from build123d import *

# Parameters (mm, degrees)
F1_DEPTH = 9.525
F3_DEPTH = 4.445


with BuildPart() as f1:
    # F0 (on Front) → F1 (new body)
    with BuildSketch(Plane.XZ):
        with BuildLine():
            ThreePointArc((-5.707243, -7.21562), (-9.19628, -0.257349), (-6.101839, 6.885154))
            ThreePointArc((-6.101839, 6.885154), (-5.88147, 7.779725), (-6.639719, 8.303058))
            Line((-6.639719, 8.303058), (-6.639719, 7.998258))
            ThreePointArc((-6.639719, 7.998258), (-6.166454, 7.671617), (-6.303998, 7.113266))
            ThreePointArc((-6.303998, 7.113266), (-9.500428, -0.284281), (-5.8674, -7.47747))
            Line((-5.8674, -7.47747), (-5.8674, -9.920767))
            Line((-5.8674, -9.920767), (-5.8674, -10.867245))
            Line((-5.8674, -10.867245), (5.8674, -10.867245))
            Line((5.8674, -10.867245), (5.8674, -7.47747))
            ThreePointArc((5.8674, -7.47747), (9.502004, -0.225537), (6.215559, 7.190673))
            ThreePointArc((6.215559, 7.190673), (6.072203, 7.750216), (6.54657, 8.079787))
            Line((6.54657, 8.079787), (6.54657, 8.384587))
            ThreePointArc((6.54657, 8.384587), (5.786557, 7.856561), (6.016236, 6.960079))
            ThreePointArc((6.016236, 6.960079), (9.197695, -0.200486), (5.707243, -7.21562))
            ThreePointArc((5.707243, -7.21562), (5.600662, -7.34845), (5.5626, -7.514445))
            Line((5.5626, -7.514445), (5.5626, -10.562445))
            Line((5.5626, -10.562445), (-5.5626, -10.562445))
            Line((-5.5626, -10.562445), (-5.5626, -9.920767))
            Line((-5.5626, -9.920767), (-5.5626, -7.514445))
            ThreePointArc((-5.5626, -7.514445), (-5.600662, -7.34845), (-5.707243, -7.21562))
        make_face()
    extrude(amount=F1_DEPTH)

    # F2 (on Right) → F3 (join, symmetric)
    with BuildSketch(Plane.YZ):
        with BuildLine():
            Line((0, -10.562445), (0, -10.867245))
            Line((0, -10.867245), (3.1623, -10.867245))
            ThreePointArc((3.1623, -10.867245), (3.476609, -10.737054), (3.6068, -10.422745))
            Line((3.6068, -10.422745), (3.6068, 3.748756))
            ThreePointArc((3.6068, 3.748756), (3.617336, 3.844964), (3.648446, 3.93661))
            Line((3.648446, 3.93661), (4.455377, 5.667079))
            Line((4.455377, 5.667079), (4.179134, 5.795893))
            Line((4.179134, 5.795893), (3.372204, 4.065424))
            ThreePointArc((3.372204, 4.065424), (3.319761, 3.910935), (3.302, 3.748756))
            Line((3.302, 3.748756), (3.302, -10.562445))
            Line((3.302, -10.562445), (0, -10.562445))
        make_face()
    extrude(amount=F3_DEPTH, both=True)

    # F4 (on Right) → F5 (revolve)
    with BuildSketch(Plane.YZ):
        with BuildLine():
            Line((3.302, -1.088245), (2.032, -1.088245))
            ThreePointArc((2.032, -1.088245), (2.374146, -2.316276), (3.302, -3.190469))
            Line((3.302, -3.190469), (3.302, -1.088245))
        make_face()
    revolve(axis=Axis((0, 2.667, -1.088245), (0, -1, 0)))


solid = f1.part
Can you work these out from the model? Positions are in its coordinate system, mm. A direction names the side the tool comes from. Give positions to 0.01 mm unless a question says otherwise; leave off trailing zeros. Loops run counter-clockwise (first coordinate to the right, second up) from the corner with the lowest first, then second, coordinate; pieces in that order, holes last. Notation, with made-up numbers: M 31.5,65 L 73.5,65 A19 ccw 73.5,102 Z; hole C 58,89 d5. An arc over 180 degrees is marked long. One line per item, written item: value. Start each with the question number.
1) Thinking about a two-plate mould opening in X: for faces 6 (the face through (0.06, 3.78, 4.94)), 7 (the face through (9.5, -4.7, -0.3)), 8 (the face through (0, -3, -10.562)), 9 (the face through (-5.867, -5, -9)), which applies, +X half, -X half, draft (parallel to the pull), parting line (faces both ways), or undercut?
2) I'm going to push flat-ended pins straight in: pin 1 (8 mm diameter, centred on y = -1.5, z = -6.5, fed in from +X); pin 2 (5.5 mm diameter, centred on x = -6.5, z = -1, fed in from +Y); pin 3 (2.5 mm diameter, centred on y = -3, z = -9, fed in from -X); pin 4 (1.3 mm diameter, centred on y = 1.5, z = -3.5, fed in from +X). Where does each tip first touch, or does it pass through?
3) If we section it at B-B, the plane z = 6.5: Write out the boundary of the cut face in (x, y) (3 decimals), and give its area (3 significant figures).
4) On a 3-axis mill with a long thin cutter (end or side, diameter ignored), from which of +Z, -Z, +X, -X, +Y, -Y can I reach the whole of each face in a straight line? I mean faces 1 (the face through (6.07, -4.7, 7.74)), 2 (the face through (-5.563, -5, -9)), 3 (the face through (-9.503, -4.696, -0.168)), 4 (the face through (0, 3.607, -3)), 5 (the face through (9.2, -4.7, -0.1)). Say none if no direction works.
5) If I drill on line 1 (X direction, y = -8.75, z = -9.5); line 2 (Z direction, x = 6.5, y = -7.75); line 3 (X direction, y = -2.5, z = 3.5), over which ranges is the centre line in solid material (lowest first)? Write a range as [from, to].
6) If we section it at A-A, the plane z = -8.75: Write out the boundary of the cut face in (x, y) (3 decimals), and give its area (3 significant figures).
7) If we section it at D-D, the plane y = -8.25: Write out the boundary of the cut face in (x, z).
Completed:
1. face 6: draft
1. face 7: +X half
1. face 8: undercut
1. face 9: -X half
2. pin 1: stops at x = 9.17
2. pin 2: stops at y = 3.61
2. pin 3: stops at x = -5.87
2. pin 4: passes through
3. outline: M -6.935,-9.525 L -6.511,-9.525 L -6.511,0 L -6.935,0 Z; M 6.511,-9.525 L 6.935,-9.525 L 6.935,0 L 6.511,0 Z
3. area: 8.08 mm^2
4. face 1: +X, +Y, -Y
4. face 2: +Z, +Y, -Y
4. face 3: -X, +Y, -Y
4. face 4: -Z, +X, -X, +Y
4. face 5: +Y, -Y
5. line 1: x = [-5.87, -5.56], [5.56, 5.87]
5. line 2: z = [-6.93, -6.51], [6.51, 6.93], [8.08, 8.38]
5. line 3: x = [-8.84, -8.51], [8.51, 8.84]
6. outline: M -5.867,-9.525 L -5.563,-9.525 L -5.563,0 L -5.867,0 Z; M -4.445,3.302 L 4.445,3.302 L 4.445,3.607 L -4.445,3.607 Z; M 5.563,-9.525 L 5.867,-9.525 L 5.867,0 L 5.563,0 Z
6. area: 8.52 mm^2
7. outline: M -6.64,8 A0.51 cw -6.3,7.11 A9.5 ccw -5.87,-7.48 L -5.87,-10.87 L 5.87,-10.87 L 5.87,-7.48 A9.5 ccw 6.22,7.19 A0.51 cw 6.55,8.08 L 6.55,8.38 A0.81 ccw 6.02,6.96 A9.2 cw 5.71,-7.22 A0.38 ccw 5.56,-7.51 L 5.56,-10.56 L -5.56,-10.56 L -5.56,-7.51 A0.38 ccw -5.71,-7.22 A9.2 cw -6.1,6.89 A0.81 ccw -6.64,8.3 Z
